Build history of the part. All positions in model axes, mm. Coordinates: 2 decimals unless noted, no trailing zeros. Loops run counter-clockwise (first coordinate to the right, second up) from the corner with the lowest first, then second, coordinate; pieces in that order, holes last. Notation, with made-up numbers: (8.5, 62) - (32.5, 62) arc R24 ccw to (32.5, 72) - close; hole circle Ø4 at (-23.5, -21). An arc over 180 degrees is marked (long way). One line per item, written item: value.
```python
from build123d import *

# Parameters (mm, degrees)
BOSS_EXTRUDE1_DEPTH = 3
SKETCH2_R           = 2.5
CUT_EXTRUDE1_DEPTH  = 3
CIRPATTERN1_COUNT   = 4


with BuildPart() as part:
    # Sketch1 → Boss-Extrude1 (new body)
    with BuildSketch(Plane.XY):
        with BuildLine():
            Line((-361, 180.5), (-361, -180.5))
            ThreePointArc((-361, -180.5), (-233.367225996, -233.367225996), (-180.5, -361))
            Line((-180.5, -361), (180.5, -361))
            ThreePointArc((180.5, -361), (233.367225996, -233.367225996), (361, -180.5))
            Line((361, -180.5), (361, 180.5))
            ThreePointArc((361, 180.5), (233.367225996, 233.367225996), (180.5, 361))
            Line((180.5, 361), (-180.5, 361))
            ThreePointArc((-180.5, 361), (-233.367225996, 233.367225996), (-361, 180.5))
        make_face()
    extrude(amount=BOSS_EXTRUDE1_DEPTH)

    # Sketch2 → Cut-Extrude1 (cut)
    with BuildSketch(Plane.XY.offset(3)):
        with Locations((-351.5, 165)):
            Circle(SKETCH2_R)
        with Locations((-351.5, 150)):
            Circle(SKETCH2_R)
        with Locations((-351.5, 135)):
            Circle(SKETCH2_R)
        with Locations((-351.5, 120)):
            Circle(SKETCH2_R)
        with Locations((-351.5, 105)):
            Circle(SKETCH2_R)
        with Locations((-351.5, 90)):
            Circle(SKETCH2_R)
        with Locations((-351.5, 75)):
            Circle(SKETCH2_R)
        with Locations((-351.5, 60)):
            Circle(SKETCH2_R)
        with Locations((-351.5, 45)):
            Circle(SKETCH2_R)
        with Locations((-351.5, 30)):
            Circle(SKETCH2_R)
        with Locations((-351.5, 15)):
            Circle(SKETCH2_R)
        with Locations((-351.5, 0)):
            Circle(SKETCH2_R)
        with Locations((-351.5, -15)):
            Circle(SKETCH2_R)
        with Locations((-351.5, -30)):
            Circle(SKETCH2_R)
        with Locations((-351.5, -165)):
            Circle(SKETCH2_R)
        with Locations((-351.5, -150)):
            Circle(SKETCH2_R)
        with Locations((-351.5, -135)):
            Circle(SKETCH2_R)
        with Locations((-351.5, -120)):
            Circle(SKETCH2_R)
        with Locations((-351.5, -45)):
            Circle(SKETCH2_R)
        with Locations((-351.5, -60)):
            Circle(SKETCH2_R)
        with Locations((-351.5, -75)):
            Circle(SKETCH2_R)
        with Locations((-351.5, -90)):
            Circle(SKETCH2_R)
        with Locations((-351.5, -105)):
            Circle(SKETCH2_R)
    cut_extrude1 = extrude(amount=-CUT_EXTRUDE1_DEPTH, mode=Mode.SUBTRACT)

    # CirPattern1: Cut-Extrude1 ×4 about axis
    cirpattern1_axis = Axis((0.379323616, 0, 0), (0, 0, 1))
    for i in range(1, CIRPATTERN1_COUNT):
        add(cut_extrude1.rotate(cirpattern1_axis, i * 360 / CIRPATTERN1_COUNT), mode=Mode.SUBTRACT)


solid = part.part
```
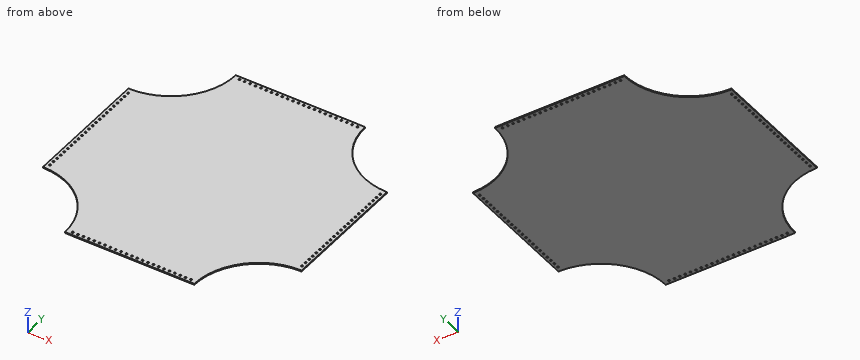
Item 1: Cut at C-C, the plane y = -281. Write the cut outline in (x, z), then the cut area to 3 significant figures.
Check result:
outline: (-199.2, 0) - (199.2, 0) - (199.2, 3) - (-199.2, 3) - close
area: 1,200 mm^2
Item 2: Probe probe 1 along Y at (x, z) = (45.5, 1.55); probe 2 along X at (y, z) = (-135, 1.5); probe 3 along X at (y, z) = (163, 1.65). List the from-to ranges inside material, lowest first. Write a range as from..to.
Check result:
probe 1: y = -361..-354.38, -349.38..349.38, 354.38..361
probe 2: x = -361..-354, -349..349.76, 354.76..361
probe 3: x = -361..-353, -350..350.76, 353.76..361
Item 3: Drop flat-ended pins along their axis: P1, Ø4.5, axis at x = -119.62, y = 351.88, coming from the +Z side; P2, Ø1.5, axis at x = 220, z = 2.5, coming from the -Y side. Give the stop position or say it passes through.
Check result:
P1: passes through
P2: stops at y = -249.25
Item 4: Cut at B-B, the plane x = 222. Write the cut outline in (y, z), then the cut area to 3 significant figures.
Check result:
outline: (-245.85, 0) - (245.85, 0) - (245.85, 3) - (-245.85, 3) - close
area: 1,480 mm^2
Item 5: Cut at A-A, the plane z = 2.2. Give the number of separate pieces and of enclosed holes in the cut face, then the cut area to 3 significant figures.
Check result:
separate pieces: 1
enclosed holes: 92
area: 417,000 mm^2
